from build123d import *

# Parameters (mm, degrees)
ESBO_O1_W                = 51
ESBO_O1_H                = 51
RESSALTO_EXTRUS_O1_DEPTH = 6
ESBO_O2_W                = 36.5
ESBO_O2_H                = 6.5
CORTE_EXTRUS_O1_DEPTH    = 4.5
ESBO_O3_R                = 2
CORTE_EXTRUS_O2_DEPTH    = 37.558172821
ESBO_O4_W                = 44
ESBO_O4_H                = 30.5
CORTE_EXTRUS_O3_DEPTH    = 4.5
FILETE1_R                = 2
CHANFRO1_SIZE            = 1
RESSALTO_EXTRUS_O2_DEPTH = 2
RESSALTO_EXTRUS_O3_REACH = 56.245


with BuildPart() as part:
    # Esboço1 → Ressalto-extrusão1 (new body)
    with BuildSketch(Plane.XY):
        Rectangle(ESBO_O1_W, ESBO_O1_H)
    extrude(amount=RESSALTO_EXTRUS_O1_DEPTH)

    # Esboço2 → Corte-extrusão1 (cut)
    with BuildSketch(Plane(origin=(0, 0, 0), x_dir=(-1, 0, 0), z_dir=(0, 0, -1))):
        with Locations((0, -19.25)):
            Rectangle(ESBO_O2_W, ESBO_O2_H)
    extrude(amount=-CORTE_EXTRUS_O1_DEPTH, mode=Mode.SUBTRACT)

    # Esboço3 → Corte-extrusão2 (cut, through all)
    with BuildSketch(Plane.XY.offset(6)):
        with Locations((0, 20.5)):
            Circle(ESBO_O3_R)
    extrude(amount=-CORTE_EXTRUS_O2_DEPTH, mode=Mode.SUBTRACT)

    # Esboço4 → Corte-extrusão3 (cut)
    with BuildSketch(Plane(origin=(0, 0, 0), x_dir=(-1, 0, 0), z_dir=(0, 0, -1))):
        with Locations((0, 1.25)):
            Rectangle(ESBO_O4_W, ESBO_O4_H)
    extrude(amount=-CORTE_EXTRUS_O3_DEPTH, mode=Mode.SUBTRACT)

    # Filete1
    filete1_edges = [part.edges().sort_by_distance(p)[0] for p in [
        (0, 25.5, 6),
    ]]
    fillet(filete1_edges, radius=FILETE1_R)

    # Chanfro1
    chanfro1_edges = [part.edges().sort_by_distance(p)[0] for p in [
        (-2, 20.5, 6),
    ]]
    chamfer(chanfro1_edges, length=CHANFRO1_SIZE - 0.0001)  # a hair under: the kernel refuses the full size

    # Esboço5 → Ressalto-extrusão2 (add)
    with BuildSketch(Plane(origin=(0, 0, 0), x_dir=(-1, 0, 0), z_dir=(0, 0, -1))):
        Polygon((-23.5, 19.5), (-21.5, 19.5), (-21.5, 21.5), (-19.5, 21.5), (-19.5, 23.5), (-23.5, 23.5), align=None)
        Polygon((21.5, 19.5), (23.5, 19.5), (23.5, 23.5), (19.5, 23.5), (19.5, 21.5), (21.5, 21.5), align=None)
    extrude(amount=RESSALTO_EXTRUS_O2_DEPTH)

    # Ressalto-extrusão3: up to this face of the body (flat: up to its plane)
    ressalto_extrus_o3_end = Plane(part.part.faces().sort_by_distance((22, 1.25, 2.25))[0])
    # Esboço6 → Ressalto-extrusão3 (add, up to the picked face)
    with BuildSketch(Plane(origin=(-22, 0, 0), x_dir=(0, 0, -1), z_dir=(1, 0, 0)), mode=Mode.PRIVATE) as ressalto_extrus_o3_sk1:
        Polygon((0, -16), (2, -14), (0, -14), align=None)
    ressalto_extrus_o3_tool1 = split(extrude(ressalto_extrus_o3_sk1.sketch, amount=RESSALTO_EXTRUS_O3_REACH, mode=Mode.PRIVATE), bisect_by=ressalto_extrus_o3_end, keep=Keep.BOTH, mode=Mode.PRIVATE)
    # Esboço6 → Ressalto-extrusão3 (add, up to the picked face)
    with BuildSketch(Plane(origin=(-22, 0, 0), x_dir=(0, 0, -1), z_dir=(1, 0, 0)), mode=Mode.PRIVATE) as ressalto_extrus_o3_sk2:
        Polygon((-4.5, -1.5), (2, -1.5), (-4.5, -4), align=None)
    ressalto_extrus_o3_tool2 = split(extrude(ressalto_extrus_o3_sk2.sketch, amount=RESSALTO_EXTRUS_O3_REACH, mode=Mode.PRIVATE), bisect_by=ressalto_extrus_o3_end, keep=Keep.BOTH, mode=Mode.PRIVATE)
    # Esboço6 → Ressalto-extrusão3 (add, up to the picked face)
    with BuildSketch(Plane(origin=(-22, 0, 0), x_dir=(0, 0, -1), z_dir=(1, 0, 0)), mode=Mode.PRIVATE) as ressalto_extrus_o3_sk3:
        Polygon((-4.5, 8.5), (2, 11), (-4.5, 11), align=None)
    ressalto_extrus_o3_tool3 = split(extrude(ressalto_extrus_o3_sk3.sketch, amount=RESSALTO_EXTRUS_O3_REACH, mode=Mode.PRIVATE), bisect_by=ressalto_extrus_o3_end, keep=Keep.BOTH, mode=Mode.PRIVATE)
    add(ressalto_extrus_o3_tool1.solids().sort_by(Axis((-22, -14.666667, -0.666667), (1, 0, 0)))[0])
    add(ressalto_extrus_o3_tool2.solids().sort_by(Axis((-22, -2.333333, 2.333333), (1, 0, 0)))[0])
    add(ressalto_extrus_o3_tool3.solids().sort_by(Axis((-22, 10.166667, 2.333333), (1, 0, 0)))[0])


solid = part.part
Build history of the part. All positions in model axes, mm. A direction names the side the tool comes from. Give positions to 0.01 mm unless a question says otherwise; leave off trailing zeros. Loops run counter-clockwise (first coordinate to the right, second up) from the corner with the lowest first, then second, coordinate; pieces in that order, holes last. Notation, with made-up numbers: (73, 21.25) -> (84, 21.25) arc R17 cw to (84, 52.25) -> close; hole circle Ø6 at (51.25, 31.5). An arc over 180 degrees is marked (long way). Answer in a Markdown table with one row per item.
Item 1: Slice it at A-A on y = 20.5. Write the cut outline in (x, z), plus the area to 3 significant figures.
Findings below:
| item | result |
|---|---|
| outline | (-25.5, 0) -> (-23.5, 0) -> (-23.5, -2) -> (-21.5, -2) -> (-21.5, 0) -> (-2, 0) -> (-2, 5) -> (-3, 6) -> (-25.5, 6) -> close; (2, 0) -> (21.5, 0) -> (21.5, -2) -> (23.5, -2) -> (23.5, 0) -> (25.5, 0) -> (25.5, 6) -> (3, 6) -> (2, 5) -> close |
| area | 289 mm² |
Item 2: Slice it at C-C on z = 1.25. Write the cut outline in (x, y).
Findings below:
| item | result |
|---|---|
| outline | (-25.5, -25.5) -> (25.5, -25.5) -> (25.5, 25.5) -> (-25.5, 25.5) -> close; hole (-22, -14) -> (22, -14) -> (22, -2.75) -> (-22, -2.75) -> close; hole (-22, -1.5) -> (22, -1.5) -> (22, 9.75) -> (-22, 9.75) -> close; hole (-22, 11) -> (22, 11) -> (22, 16.5) -> (-22, 16.5) -> close; hole (-18.25, -22.5) -> (18.25, -22.5) -> (18.25, -16) -> (-18.25, -16) -> close; hole circle Ø4 at (0, 20.5) |
Item 3: Probe line 1 along Y through (x, z) = (-1.5, -1.5); line 2 along Y through (x, z) = (-10.5, 3); line 3 along Y through (x, z) = (3.5, -0.5). List the from-to ranges inside material, lowest first. Write a range as [from, to].
Findings below:
| item | result |
|---|---|
| line 1 | y = [-14.5, -14], [-1.69, -1.5], [10.81, 11] |
| line 2 | y = [-25.5, -22.5], [-16, -14], [-3.42, -1.5], [9.08, 11], [16.5, 25.5] |
| line 3 | y = [-15.5, -14], [-2.08, -1.5], [10.42, 11] |
Item 4: Tool access for faces 4 (the cylindrical face through (-0.26, 22.483, 2.535)), 5 (the flat face through (-0.31, -2.73, 1.2)), 6 (the flat face through (-22, 19.5, -1)), 7 (the flat face through (19.5, 22, -1)), 8 (the flat face through (22, 22, -2)): list every direction of +Z, -Z, +X, -X, +Y, -Y with a clear straight run to the whole face (end or side of a thin tool).
Findings below:
| item | result |
|---|---|
| face 4 | +Z, -Z |
| face 5 | -Z |
| face 6 | -Z, +X, -X |
| face 7 | -Z, +Y |
| face 8 | -Z, +X, -X, +Y, -Y |
Item 5: Mould opens along X. For faces 1 (the flat face through (-23.5, 21, -1)), 2 (the flat face through (-19.5, 23, -1)), 3 (the flat face through (21, 23.5, -1)) say: pulls with the +X half, pulls with the -X half, needs draft (parallel to the pull), parting line crosses it, or undercut.
Findings below:
| item | result |
|---|---|
| face 1 | pulls with the -X half |
| face 2 | undercut |
| face 3 | needs draft |
Item 6: Slice it at D-D on y = 3. Write the cut outline in (x, z).
Findings below:
| item | result |
|---|---|
| outline | (-25.5, 0) -> (-22, 0) -> (-22, 4.5) -> (22, 4.5) -> (22, 0) -> (25.5, 0) -> (25.5, 6) -> (-25.5, 6) -> close |
Item 7: Flat gauge pins, fed straight in: P1, Ø4.5, axis at x = 6.5, y = 15, coming from the -Z side; P2, Ø2, axis at x = -2, y = -20.5, coming from the -Z side; P3, Ø2, axis at x = -20, z = -1.5, coming from the -Y side. Where does each tip first touch, or does it go through?
Findings below:
| item | result |
|---|---|
| P1 | stops at z = 0 |
| P2 | stops at z = 4.5 |
| P3 | stops at y = -15.5 |
